Geometry: see drawing. Coordinates: mm, zero at the bounding-box minimum. Give positions to 0.01 mm unless a question says otherwise; leave off trailing zeros. Loops run counter-clockwise (first coordinate to the right, second up) from the corner with the lowest first, then second, coordinate; pieces in that order, holes last. Notation, with made-up numbers: (-25, 11.25) -> (11, 11.25) arc R9 cw to (11, 16.25) -> close; hole circle Ø3 at (-3, 87). An arc over 180 degrees is marked (long way). One line per question, with ' | ' between items.
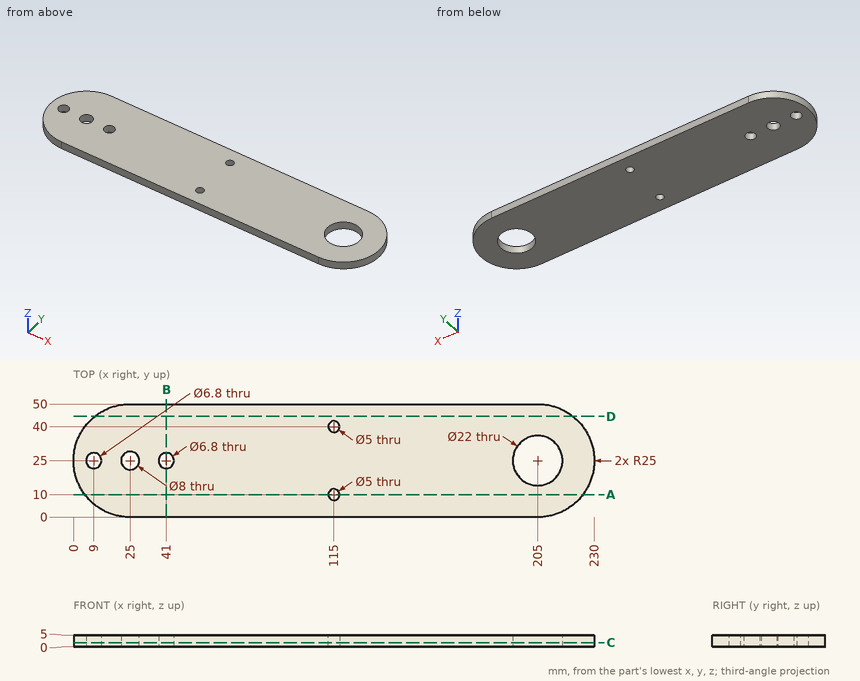
1. Ray query, line 1 along Y through (x, z) = (115, 2.55); line 2 along X through (y, z) = (23.5, 0.45); line 3 along X through (y, z) = (23, 3.85). Return the intervals inside material, ascending. Write a range as from..to.
Determined:
line 1: y = 0..7.5, 12.5..37.5, 42.5..50 | line 2: x = 0.05..5.95, 12.05..21.29, 28.71..37.95, 44.05..194.1, 215.9..229.95 | line 3: x = 0.08..6.25, 11.75..21.54, 28.46..38.25, 43.75..194.18, 215.82..229.92
2. Section query B-B (x = 41). Output: boundary loops of the cut face in (y, z).
Determined:
outline: (0, 0) -> (21.6, 0) -> (21.6, 5) -> (0, 5) -> close; (28.4, 0) -> (50, 0) -> (50, 5) -> (28.4, 5) -> close
3. Section query C-C (z = 1.7). Output: boundary loops of the cut face in (x, y).
Determined:
outline: (25, 0) -> (205, 0) arc R25 ccw to (205, 50) -> (25, 50) arc R25 ccw to start; hole circle Ø6.8 at (9, 25); hole circle Ø8 at (25, 25); hole circle Ø6.8 at (41, 25); hole circle Ø5 at (115, 10); hole circle Ø5 at (115, 40); hole circle Ø22 at (205, 25)
4. Section query A-A (y = 10). Output: boundary loops of the cut face in (x, z).
Determined:
outline: (5, 0) -> (112.5, 0) -> (112.5, 5) -> (5, 5) -> close; (117.5, 0) -> (225, 0) -> (225, 5) -> (117.5, 5) -> close
5. Section query D-D (y = 44.5). Output: boundary loops of the cut face in (x, z), then the cut area to 3 significant figures.
Determined:
outline: (9.36, 0) -> (220.64, 0) -> (220.64, 5) -> (9.36, 5) -> close | area: 1,060 mm2
6. Pin query (flat end, axial travel): P1, Ø1, axis at y = 9, z = 3.5, coming from the +X side; P2, Ø3, axis at y = 14, z = 0.5, coming from the -X side; P3, Ø1.5, axis at y = 43.5, z = 0.5, coming from the +X side. Return the tip coordinate at first contact, or that it passes through.
Determined:
P1: stops at x = 224.62 | P2: stops at x = 1.88 | P3: stops at x = 222.61
